Read the model definition and answer for the solid it produces. Units are mm, in the model's axes. A direction names the side the tool comes from. Coordinates: 2 decimals unless noted, no trailing zeros. Write each loop counter-clockwise with the first axis right and the second up, starting at its lowest first coordinate (ties: lowest second). Pieces come first, ordered by that corner, then holes. Notation, with made-up numbers: (13, 55.5) - (29, 55.5) arc R22 ccw to (29, 67.5) - close; hole circle Ø1 at (-21, -6). An arc over 180 degrees is marked (long way). Return JSON: item names as keys, results as strings.
```python
from build123d import *

# Parameters (mm, degrees)
BOSS_EXTRUDE1_DEPTH = 1
BOSS_EXTRUDE2_DEPTH = 1
BOSS_EXTRUDE3_DEPTH = 1


with BuildPart() as part:
    # Sketch1 → Boss-Extrude1 (new body)
    with BuildSketch(Plane.XY):
        with BuildLine():
            Line((30.054563517, 47.732233047), (40.661165235, 58.338834765))
            ThreePointArc((40.661165235, 58.338834765), (58.338834765, 58.338834765), (58.338834765, 40.661165235))
            Line((58.338834765, 40.661165235), (47.732233047, 30.054563517))
            Line((47.732233047, 30.054563517), (47.732233047, 0))
            Line((47.732233047, 0), (0, 0))
            Line((0, 0), (0, 47.732233047))
            Line((0, 47.732233047), (30.054563517, 47.732233047))
        make_face()
    extrude(amount=-BOSS_EXTRUDE1_DEPTH)

    # Sketch2 → Boss-Extrude2 (add)
    with BuildSketch(Plane(origin=(0, 0, 0), x_dir=(0, 0, -1), z_dir=(1, 0, 0))):
        with BuildLine():
            Line((30.054563517, 47.732233047), (40.661165235, 58.338834765))
            ThreePointArc((40.661165235, 58.338834765), (58.338834765, 58.338834765), (58.338834765, 40.661165235))
            Line((58.338834765, 40.661165235), (47.732233047, 30.054563517))
            Line((47.732233047, 30.054563517), (47.732233047, 0))
            Line((47.732233047, 0), (0, 0))
            Line((0, 0), (0, 47.732233047))
            Line((0, 47.732233047), (30.054563517, 47.732233047))
        make_face()
    extrude(amount=BOSS_EXTRUDE2_DEPTH)

    # Sketch3 → Boss-Extrude3 (add)
    with BuildSketch(Plane(origin=(0, 0, 0), x_dir=(1, 0, 0), z_dir=(0, 1, 0))):
        with BuildLine():
            Line((30.054563517, 47.732233047), (40.661165235, 58.338834765))
            ThreePointArc((40.661165235, 58.338834765), (58.338834765, 58.338834765), (58.338834765, 40.661165235))
            Line((58.338834765, 40.661165235), (47.732233047, 30.054563517))
            Line((47.732233047, 30.054563517), (47.732233047, 0))
            Line((47.732233047, 0), (0, 0))
            Line((0, 0), (0, 47.732233047))
            Line((0, 47.732233047), (30.054563517, 47.732233047))
        make_face()
    extrude(amount=BOSS_EXTRUDE3_DEPTH)


solid = part.part
```
(1) A cutting plane is placed at B-B (x = 21). Determine the outline of the cut face in (y, z), and give its area (3 significant figures).
Answer:
{"outline": "(0, -47.73) - (1, -47.73) - (1, -1) - (47.73, -1) - (47.73, 0) - (0, 0) - close", "area": "94.5 mm²"}
(2) A cutting plane is placed at A-A (y = 49.5). Determine the outline of the cut face in (x, z), and give its area (3 significant figures).
Answer:
{"outline": "(0, -62) - (1, -62) - (1, -31.82) - (0, -31.82) - close; (31.82, -1) - (62, -1) - (62, 0) - (31.82, 0) - close", "area": "60.4 mm²"}
(3) Straight lines are drawn through the part: line 1 (Z direction, x = 7.5, y = 37.5); line 2 (Y direction, x = 5.5, z = -42.5). For each, find the intervals that lie inside material, in ascending order. Write a range as from..to.
Answer:
{"line 1": "-1..0", "line 2": "0..1"}
(4) A cutting plane is placed at C-C (z = -49.5). Determine the outline of the cut face in (x, y), and give its area (3 significant figures).
Answer:
{"outline": "(0, 31.82) - (1, 31.82) - (1, 62) - (0, 62) - close; (31.82, 0) - (62, 0) - (62, 1) - (31.82, 1) - close", "area": "60.4 mm²"}
(5) Flat-ended cylindrical pins translate along their axes: P1, Ø8, axis at x = 22.5, z = -34, coming from the +Y side; P2, Ø12, axis at x = 10.5, y = 26.5, coming from the -Z side; P3, Ø18.5, axis at y = 38.5, z = -22, coming from the +X side. Find the tip coordinate at first contact, or state that the pin passes through.
Answer:
{"P1": "y = 1", "P2": "z = -1", "P3": "x = 1"}
(6) Which of the six approach directions +Z, -Z, +X, -X, +Y, -Y give full straight-line access (tool end or side, diameter ignored) to faces 1 (the face through (1, 32, -32)), 2 (the face through (0.5, 8.3, -47.732)), 3 (the face through (8.3, 47.732, -0.5)), 4 (the face through (35.28, 52.96, -0.49)), 5 (the face through (47.732, 8.3, -0.6))?
Answer:
{"face 1": "-Z, +X, +Y", "face 2": "-Z, -X, -Y", "face 3": "+Z, -X, +Y", "face 4": "+Z, -Z, -X, +Y", "face 5": "+Z, +X, -Y"}
